Work out the finished part from the listing and answer in its coordinate system (mm). Coordinates: 2 decimals unless noted, no trailing zeros. Loops run counter-clockwise (first coordinate to the right, second up) from the corner with the lowest first, then second, coordinate; pieces in that order, holes last. Notation, with made-up numbers: (-8.75, 11) -> (3.25, 11) arc R12 ccw to (3.25, 29) -> close; hole circle Ø10 at (48, 58). An arc over 180 degrees is marked (long way). Answer as CSV lines item,"result".
```python
from build123d import *

# Parameters (mm, degrees)
BOSS_EXTRUDE1_DEPTH = 24
CUT_EXTRUDE1_DEPTH  = 2.5
SKETCH3_R           = 1
CUT_EXTRUDE3_DEPTH  = 8.5
CUT_EXTRUDE4_START  = 5
SKETCH4_R           = 2.55
CUT_EXTRUDE4_DEPTH  = 5
SKETCH5_R           = 2.55
CUT_EXTRUDE5_DEPTH  = 10


with BuildPart() as part:
    # Sketch1 → Boss-Extrude1 (new body)
    with BuildSketch(Plane(origin=(0, 0, 0), x_dir=(1, 0, 0), z_dir=(0, 1, 0))):
        with BuildLine():
            ThreePointArc((0, -3), (-3, 0), (0, 3))
            Line((0, 3), (0, 4.5))
            ThreePointArc((0, 4.5), (-4.5, 0), (0, -4.5))
            Line((0, -4.5), (0, -3))
        make_face()
        with BuildLine():
            Line((0, 4.5), (0, 3))
            ThreePointArc((0, 3), (2.121320344, 2.121320344), (3, 0))
            ThreePointArc((3, 0), (2.121320344, -2.121320344), (0, -3))
            Line((0, -3), (0, -4.5))
            ThreePointArc((0, -4.5), (3.181980515, -3.181980515), (4.5, 0))
            ThreePointArc((4.5, 0), (3.181980515, 3.181980515), (0, 4.5))
        make_face()
        with BuildLine():
            Line((10, 4.5), (0, 4.5))
            ThreePointArc((0, 4.5), (3.181980515, 3.181980515), (4.5, 0))
            ThreePointArc((4.5, 0), (3.181980515, -3.181980515), (0, -4.5))
            Line((0, -4.5), (10, -4.5))
            Line((10, -4.5), (10, 4.5))
        make_face()
    extrude(amount=BOSS_EXTRUDE1_DEPTH)

    # Sketch2 → Cut-Extrude1 (cut)
    with BuildSketch(Plane(origin=(10, 0, 0), x_dir=(0, 0, -1), z_dir=(1, 0, 0))):
        with BuildLine():
            ThreePointArc((2.55, 12), (1.803122292, 13.803122292), (0, 14.55))
            Line((0, 14.55), (0, 9.45))
            ThreePointArc((0, 9.45), (1.803122292, 10.196877708), (2.55, 12))
        make_face()
        with BuildLine():
            Line((0, 9.45), (0, 14.55))
            ThreePointArc((0, 14.55), (-2.55, 12), (0, 9.45))
        make_face()
    extrude(amount=-CUT_EXTRUDE1_DEPTH, mode=Mode.SUBTRACT)

    # Sketch3 → Cut-Extrude3 (cut)
    with BuildSketch(Plane(origin=(7.5, 0, 0), x_dir=(0, 0, -1), z_dir=(1, 0, 0))):
        with Locations((0, 12)):
            Circle(SKETCH3_R)
    extrude(amount=-CUT_EXTRUDE3_DEPTH, mode=Mode.SUBTRACT)

    # Sketch4 → Cut-Extrude4 (cut)
    with BuildSketch(Plane(origin=(0.5, 0, 0), x_dir=(0, 0, -1), z_dir=(1, 0, 0)).offset(CUT_EXTRUDE4_START)):
        with Locations((0, 12)):
            Circle(SKETCH4_R)
    extrude(amount=-CUT_EXTRUDE4_DEPTH, mode=Mode.SUBTRACT)

    # Sketch5 → Cut-Extrude5 (cut)
    with BuildSketch(Plane(origin=(0.5, 0, 0), x_dir=(0, 0, -1), z_dir=(1, 0, 0))):
        with Locations((0, 12)):
            Circle(SKETCH5_R)
    extrude(amount=-CUT_EXTRUDE5_DEPTH, mode=Mode.SUBTRACT)


solid = part.part
```
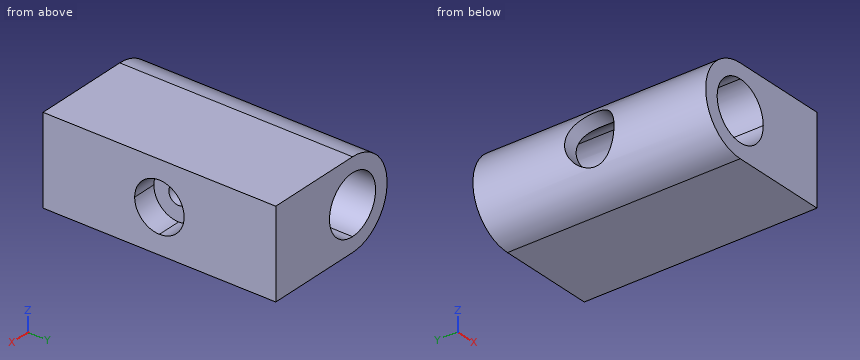
(1) Flat-ended cylindrical pins translate along their axes: pin 1 Ø1 at (y, z) = (3, 3.5) entering from -X; pin 2 Ø4 at (y, z) = (11.5, 1) entering from -X; pin 3 Ø1 at (x, z) = (1.5, -1.5) entering from +Y; pin 4 Ø3 at (y, z) = (12, 0) entering from -X. Find the tip coordinate at first contact, or state that the pin passes through.
Computed values:
pin 1,"x = -3.35"
pin 2,"x = -4.45"
pin 3,"through"
pin 4,"x = 5.5"
(2) A cutting plane is placed at D-D, the plane x = -1. Write down the section's boundary in (y, z).
Computed values:
outline,"(0, -4.39) -> (24, -4.39) -> (24, -2.83) -> (0, -2.83) -> close; (0, 2.83) -> (24, 2.83) -> (24, 4.39) -> (0, 4.39) -> close"
(3) A cutting plane is placed at A-A, the plane x = 5. Write down the section's boundary in (y, z).
Computed values:
outline,"(0, -4.5) -> (24, -4.5) -> (24, 4.5) -> (0, 4.5) -> close; hole circle Ø5.1 at (12, 0)"
(4) A cutting plane is placed at C-C, the plane z = -1.25. Write down the section's boundary in (x, y).
Computed values:
outline,"(-4.32, 0) -> (-2.73, 0) -> (-2.73, 9.78) -> (-4.32, 9.78) -> close; (-4.32, 14.22) -> (-2.73, 14.22) -> (-2.73, 24) -> (-4.32, 24) -> close; (2.73, 0) -> (10, 0) -> (10, 9.78) -> (7.5, 9.78) -> (7.5, 14.22) -> (10, 14.22) -> (10, 24) -> (2.73, 24) -> (2.73, 14.22) -> (5.5, 14.22) -> (5.5, 9.78) -> (2.73, 9.78) -> close"
(5) Consider line 1 along Y through (x, z) = (4.35, 0); line 2 along X through (y, z) = (22.5, 0); line 3 along Y through (x, z) = (6.8, 0). Determine where each line is inside the solid, lowest interval first.
Computed values:
line 1,"0 to 9.45, 14.55 to 24"
line 2,"-4.5 to -3, 3 to 10"
line 3,"0 to 11, 13 to 24"
(6) A cutting plane is placed at B-B, the plane y = 22.5. Write down the section's boundary in (x, z), and give its area (3 significant figures).
Computed values:
outline,"(0, -4.5) -> (10, -4.5) -> (10, 4.5) -> (0, 4.5) arc R4.5 ccw to start; hole circle Ø6 at (0, 0)"
area,"93.5 mm2"
